Could you check a few things on this model? Use its own coordinates, in mm. A direction names the side the tool comes from. Give positions to 0.01 mm unless a question says otherwise; leave off trailing zeros. Order: outer loops, then holes, each group sorted by start corner. A loop starts at its lowest first (then second) coordinate and runs counter-clockwise, first axis right, second up. Notation, with made-up numbers: M 43,33 L 58,33 A20 cw 58,72 Z; hole C 59,-17 d4. An arc over 180 degrees is marked long. Use a Markdown table: item, result. Add a question column.
Item 1: If I drill on L1, parallel to X at y = 0.75, z = -15; L2, parallel to Y at x = -4.5, z = -14.25, over which ranges is the centre line in solid material (lowest first)? Write a range as from..to.
Item 2: Suppose I cut it at B-B on y = 1. Write out the boundary of the cut face in (x, z).
Item 3: For faces 5 (the face through (-6, 0.3, -8)), 6 (the face through (6, 0.3, -8)), 7 (the face through (1, 1.9, -8)), which set-ups out of +Z, -Z, +X, -X, +Y, -Y let a thin tool reach every point of the face, with its end or its side?
Item 4: I'm going to push flat-ended pins straight in: pin 1 Ø3 at (x, z) = (-5.5, -8) entering from +Y; pin 2 Ø0.6 at (y, z) = (1.5, -8) entering from -X; pin 3 Ø1 at (y, z) = (1, -10.5) entering from +X. Where does each tip first touch, or does it pass through?
Item 5: If we mould it in two halves opening along X, with no side actions, what happens to faces 1 (the face through (0, 0, -8)), 2 (the face through (1.35, 1, -8)), 3 (the face through (-0.35, 1, -8)), 4 (the face through (0.35, 1, -8))? For each: released by +X, released by -X, zero draft, split by the parting line, or undercut.
Item 6: Suppose I cut it at A-A on z = -12. Write out the boundary of the cut face in (x, y).
Item 7: Suppose I cut it at D-D on x = 5. Write out the boundary of the cut face in (y, z), plus the area to 3 significant figures.
Item 8: Suppose I cut it at C-C on z = -3.25. Write out the boundary of the cut face in (x, y), plus the area to 3 significant figures.
from build123d import *

# Parameters (mm, degrees)
SKETCH1_W           = 9.89
SKETCH1_H           = 4.79
SKETCH1_H_2         = 0.01
SKETCH1_W_2         = 0.01
SKETCH1_H_3         = 10.99
SKETCH1_W_3         = 0.29
BOSS_EXTRUDE1_DEPTH = 0.3
SKETCH2_W           = 1
SKETCH2_H           = 15.79
BOSS_EXTRUDE2_DEPTH = 1.6


with BuildPart() as part:
    # Sketch1 → Boss-Extrude1 (new body)
    with BuildSketch(Plane(origin=(0, 0, 0), x_dir=(1, 0, 0), z_dir=(0, 1, 0))):
        with Locations((-5.295, 13.395)):
            Rectangle(SKETCH1_W, SKETCH1_H)
        with Locations((5.295, 13.395)):
            Rectangle(SKETCH1_W, SKETCH1_H)
        with Locations((-5.295, 10.995)):
            Rectangle(SKETCH1_W, SKETCH1_H_2)
        with Locations((5.295, 10.995)):
            Rectangle(SKETCH1_W, SKETCH1_H_2)
        Polygon((-0.35, 11), (-0.35, 10.99), (0.35, 10.99), (0.35, 11), (0.34, 11), (-0.34, 11), align=None)
        Polygon((-10.24, 10.99), (-10.24, 0), (10.24, 0), (10.24, 10.99), (0.35, 10.99), (-0.35, 10.99), align=None)
        with Locations((-10.245, 5.495)):
            Rectangle(SKETCH1_W_2, SKETCH1_H_3)
        with Locations((-10.395, 5.495)):
            Rectangle(SKETCH1_W_3, SKETCH1_H_3)
        with Locations((10.395, 5.495)):
            Rectangle(SKETCH1_W_3, SKETCH1_H_3)
        with Locations((10.245, 5.495)):
            Rectangle(SKETCH1_W_2, SKETCH1_H_3)
    extrude(amount=BOSS_EXTRUDE1_DEPTH)

    # Sketch2 → Boss-Extrude2 (add)
    with BuildSketch(Plane(origin=(0, 0.3, 0), x_dir=(1, 0, 0), z_dir=(0, 1, 0))):
        with Locations((-0.85, 7.895)):
            Rectangle(SKETCH2_W, SKETCH2_H)
        with Locations((0.85, 7.895)):
            Rectangle(SKETCH2_W, SKETCH2_H)
    extrude(amount=BOSS_EXTRUDE2_DEPTH)


solid = part.part
Findings below:
| question | item | result |
|---|---|---|
| 1 | L1 | x = -1.35..-0.35, 0.35..1.35 |
| 1 | L2 | y = 0..0.3 |
| 2 | outline | M -1.35,-15.79 L -0.35,-15.79 L -0.35,0 L -1.35,0 Z; M 0.35,-15.79 L 1.35,-15.79 L 1.35,0 L 0.35,0 Z |
| 3 | face 5 | +Z, -Z, -X, +Y |
| 3 | face 6 | +Z, -Z, +X, +Y |
| 3 | face 7 | +Z, -Z, +X, -X, +Y |
| 4 | pin 1 | stops at y = 0.3 |
| 4 | pin 2 | stops at x = -1.35 |
| 4 | pin 3 | stops at x = 1.35 |
| 5 | face 1 | zero draft |
| 5 | face 2 | released by +X |
| 5 | face 3 | undercut |
| 5 | face 4 | undercut |
| 6 | outline | M -10.24,0 L -0.35,0 L -0.35,1.9 L -1.35,1.9 L -1.35,0.3 L -10.24,0.3 Z; M 0.35,0 L 10.24,0 L 10.24,0.3 L 1.35,0.3 L 1.35,1.9 L 0.35,1.9 Z |
| 7 | outline | M 0,-15.79 L 0.3,-15.79 L 0.3,0 L 0,0 Z |
| 7 | area | 4.74 mm^2 |
| 8 | outline | M -10.54,0 L 10.54,0 L 10.54,0.3 L 1.35,0.3 L 1.35,1.9 L 0.35,1.9 L 0.35,0.3 L -0.35,0.3 L -0.35,1.9 L -1.35,1.9 L -1.35,0.3 L -10.54,0.3 Z |
| 8 | area | 9.52 mm^2 |
